Part model, mm, in its own coordinate system. Face numbers are marked on the shaded views. A direction names the side the tool comes from. Round coordinates to 2 decimals unless told otherwise and drop trailing zeros. Loops run counter-clockwise (first coordinate to the right, second up) from the corner with the lowest first, then second, coordinate; pieces in that order, holes last. Notation, with made-up numbers: (-15, -37.75) -> (-3, -37.75) arc R12 cw to (-3, -32.75) -> close; hole circle Ø9 at (76.5, -28.75). An arc over 180 degrees is marked (long way). Use a Markdown table: item, result. Add a question column.
Item 1: Cut at A-A, the plane z = -12. List the corners of the cut face in (x, y) (3 decimals), plus the area to 3 significant figures.
Item 2: Which spindle directions (+Z, -Z, +X, -X, +Y, -Y) get a long thin tool onto all of the face, cutting with end or side? Do the marked faces 1 and 2. Say none if no direction does.
Item 3: Cut at C-C, the plane x = 0. List the corners of the cut face in (y, z) (3 decimals).
Item 4: Probe line 1 (X direction, y = 11, z = 11) (3 decimals); line 2 (Z direction, x = 0, y = 23.25) (3 decimals). List the from-to ranges inside material, lowest first. Write a range as [from, to].
Item 5: Cut at B-B, the plane y = 19.05. List the corners of the cut face in (x, z) (3 decimals).
Item 6: Two-plate mould, pull along X, no slides. Class the marked faces 3, 4 and 5: pulls with the +X half, pulls with the -X half, needs draft (parallel to the pull), parting line crosses it, or undercut.
Item 7: Cut at D-D, the plane z = 16.5. List the corners of the cut face in (x, y).
Item 8: Flat gauge pin, fed straight in: pin 1 (8 mm diameter, centred on x = -10, y = 21.5, fed in from -Z) (3 decimals). Where does the tip first touch, or does it go through?
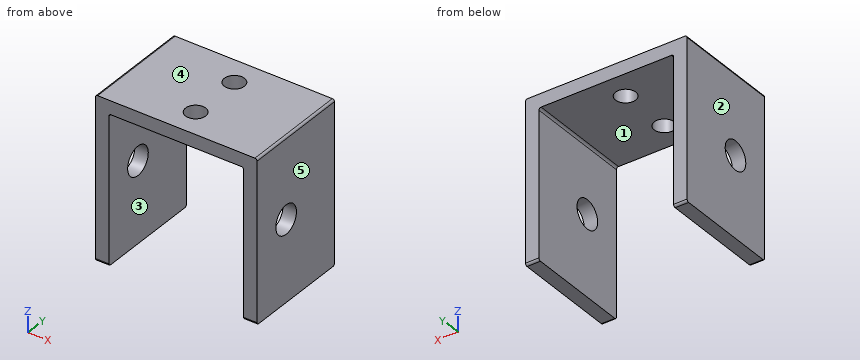
```python
from build123d import *

# Parameters (mm, degrees)
BOSS_EXTRUDE1_DEPTH            = 25.4
F_1_4_CLEARANCE_HOLE1_D        = 6.7564
F_3_16_0_1875_DIAMETER_HOLE1_D = 4.7625
FILLET1_R                      = 0.508


with BuildPart() as part:
    # Sketch1 → Boss-Extrude1 (new body)
    with BuildSketch(Plane(origin=(0, 0, 0), x_dir=(1, 0, 0), z_dir=(0, 1, 0))):
        Polygon((-15.875, 19.05), (-15.875, -15.875), (15.875, -15.875), (15.875, 19.05), (19.05, 19.05), (19.05, -19.05), (-19.05, -19.05), (-19.05, 19.05), align=None)
    extrude(amount=BOSS_EXTRUDE1_DEPTH)

    # 1/4 Clearance Hole1 (through all)
    with Locations(Plane(origin=(-19.05, 0, 0), x_dir=(0, 0, -1), z_dir=(-1, 0, 0))):
        with Locations((-0.00254, -9.525)):
            Hole(F_1_4_CLEARANCE_HOLE1_D / 2)

    # 3/16 (0.1875) Diameter Hole1 (through all)
    with Locations(Plane(origin=(0, 0, 15.875), x_dir=(-1, 0, 0), z_dir=(0, 0, -1))):
        with Locations((0, 6.35), (0, 19.05)):
            Hole(F_3_16_0_1875_DIAMETER_HOLE1_D / 2)

    # Fillet1
    fillet1_edges = [part.edges().sort_by_distance(p)[0] for p in [
        (17.4625, 0, -19.05),
        (19.05, 12.7, 19.05),
        (-19.05, 12.7, 19.05),
        (-15.875, 12.7, 15.875),
        (15.875, 12.7, 15.875),
        (-17.4625, 25.4, -19.05),
        (17.4625, 25.4, -19.05),
        (-17.4625, 0, -19.05),
    ]]
    fillet(fillet1_edges, radius=FILLET1_R)


solid = part.part
```
A:
| question | item | result |
|---|---|---|
| 1 | outline | (-19.05, 0) -> (-15.875, 0) -> (-15.875, 25.4) -> (-19.05, 25.4) -> close; (15.875, 0) -> (19.05, 0) -> (19.05, 25.4) -> (15.875, 25.4) -> close |
| 1 | area | 161 mm^2 |
| 2 | face 1 | -Z, +Y, -Y |
| 2 | face 2 | +Z, -Z, -X, +Y, -Y |
| 3 | outline | (0, 15.875) -> (3.969, 15.875) -> (3.969, 19.05) -> (0, 19.05) -> close; (8.731, 15.875) -> (16.669, 15.875) -> (16.669, 19.05) -> (8.731, 19.05) -> close; (21.431, 15.875) -> (25.4, 15.875) -> (25.4, 19.05) -> (21.431, 19.05) -> close |
| 4 | line 1 | x = [-19.05, -15.875], [15.875, 19.05] |
| 4 | line 2 | z = [15.875, 19.05] |
| 5 | outline | (-19.05, -19.05) -> (-15.875, -19.05) -> (-15.875, 15.367) arc R0.508 cw to (-15.367, 15.875) -> (-2.381, 15.875) -> (-2.381, 19.05) -> (-18.542, 19.05) arc R0.508 ccw to (-19.05, 18.542) -> close; (2.381, 15.875) -> (15.367, 15.875) arc R0.508 cw to (15.875, 15.367) -> (15.875, -19.05) -> (19.05, -19.05) -> (19.05, 18.542) arc R0.508 ccw to (18.542, 19.05) -> (2.381, 19.05) -> close |
| 6 | face 3 | undercut |
| 6 | face 4 | needs draft |
| 6 | face 5 | pulls with the +X half |
| 7 | outline | (-19.05, 0) -> (19.05, 0) -> (19.05, 25.4) -> (-19.05, 25.4) -> close; hole circle Ø4.76 at (0, 6.35); hole circle Ø4.76 at (0, 19.05) |
| 8 | pin 1 | stops at z = 15.875 |
